from build123d import *

# Parameters (mm, degrees)
BOSS_EXTRUDE1_DEPTH = 9
FILLET1_R           = 3
FILLET2_R           = 2
CUT_EXTRUDE1_REACH  = 68.828
SKETCH2_R           = 2
DRAFT1_START        = 6.699702971
DRAFT1_OUTLINE_W    = 84
DRAFT1_OUTLINE_H    = 55
DRAFT1_DEPTH        = 4.532098623


# Read off the part's stored shape, not the designer's step: Draft1
with BuildPart() as part:
    # Sketch1 → Boss-Extrude1 (new body)
    # profile 1 of 4: a face of its own
    with BuildSketch(Plane(origin=(0, 0, 0), x_dir=(1, 0, 0), z_dir=(0, 1, 0))):
        Polygon((26, 26), (-26, 26), (-26, -22), (-41, -22), (-41, -26), (-26, -26), (26, -26), (41, -26), (41, -22), (26, -22), align=None)
        Polygon((-22, -19.632135629), (-22, 22), (-2.603209536, 22), (-1.5, 22), (-1.5, 19.632135629), (-1.5, -22), (-20.896790464, -22), (-22, -22), align=None, mode=Mode.SUBTRACT)
        Polygon((1.5, 19.632135629), (1.5, 22), (2.603209536, 22), (22, 22), (22, -19.632135629), (22, -22), (20.896790464, -22), (1.5, -22), align=None, mode=Mode.SUBTRACT)
    # profile 2 of 4: a face of its own
    with BuildSketch(Plane(origin=(0, 0, 0), x_dir=(1, 0, 0), z_dir=(0, 1, 0))):
        Polygon((26, 26), (-26, 26), (-26, -22), (-41, -22), (-41, -26), (-26, -26), (26, -26), (41, -26), (41, -22), (26, -22), align=None)
        Polygon((-22, -19.632135629), (-22, 22), (-2.603209536, 22), (-1.5, 22), (-1.5, 19.632135629), (-1.5, -22), (-20.896790464, -22), (-22, -22), align=None, mode=Mode.SUBTRACT)
        Polygon((1.5, 19.632135629), (1.5, 22), (2.603209536, 22), (22, 22), (22, -19.632135629), (22, -22), (20.896790464, -22), (1.5, -22), align=None, mode=Mode.SUBTRACT)
    # profile 3 of 4: a face of its own
    with BuildSketch(Plane(origin=(0, 0, 0), x_dir=(1, 0, 0), z_dir=(0, 1, 0))):
        Polygon((-1.5, 22), (-2.603209536, 22), (-22, -19.632135629), (-22, -22), (-20.896790464, -22), (-1.5, 19.632135629), align=None)
    # profile 4 of 4: a face of its own
    with BuildSketch(Plane(origin=(0, 0, 0), x_dir=(1, 0, 0), z_dir=(0, 1, 0))):
        Polygon((2.603209536, 22), (1.5, 22), (1.5, 19.632135629), (20.896790464, -22), (22, -22), (22, -19.632135629), align=None)
    extrude(amount=BOSS_EXTRUDE1_DEPTH)

    # Fillet1
    fillet1_edges = [part.edges().sort_by_distance(p)[0] for p in [
        (-26, 4.5, 22),
        (26, 4.5, 22),
        (22, 4.5, -22),
        (2.603209536, 4.5, -22),
        (-2.603209536, 4.5, -22),
        (-22, 4.5, -22),
        (20.896790464, 4.5, 22),
        (1.5, 4.5, 22),
        (-20.896790464, 4.5, 22),
        (-1.5, 4.5, 22),
    ]]
    fillet(fillet1_edges, radius=FILLET1_R)

    # Fillet2
    fillet2_edges = [part.edges().sort_by_distance(p)[0] for p in [
        (-26, 4.5, -26),
        (26, 4.5, -26),
        (41, 4.5, 26),
        (41, 4.5, 22),
        (-41, 4.5, 22),
        (-41, 4.5, 26),
    ]]
    fillet(fillet2_edges, radius=FILLET2_R - 0.0001)  # a hair under: the kernel refuses the full size

    # Sketch2 → Cut-Extrude1 (cut, up to next)
    with BuildSketch(Plane(origin=(0, 0, -26), x_dir=(-1, 0, 0), z_dir=(0, 0, -1)), mode=Mode.PRIVATE) as cut_extrude1_sk1:
        with Locations((-13, 4.5)):
            Circle(SKETCH2_R)
    cut_extrude1_tool1 = extrude(cut_extrude1_sk1.sketch, amount=-CUT_EXTRUDE1_REACH, mode=Mode.PRIVATE) & part.part
    # Sketch2 → Cut-Extrude1 (cut, up to next)
    with BuildSketch(Plane(origin=(0, 0, -26), x_dir=(-1, 0, 0), z_dir=(0, 0, -1)), mode=Mode.PRIVATE) as cut_extrude1_sk2:
        with Locations((13, 4.5)):
            Circle(SKETCH2_R)
    cut_extrude1_tool2 = extrude(cut_extrude1_sk2.sketch, amount=-CUT_EXTRUDE1_REACH, mode=Mode.PRIVATE) & part.part
    add(cut_extrude1_tool1.solids().sort_by_distance((13, 4.5, -26))[0], mode=Mode.SUBTRACT)
    add(cut_extrude1_tool2.solids().sort_by_distance((-13, 4.5, -26))[0], mode=Mode.SUBTRACT)

    # Draft1 outline → Draft1 (cut)
    with BuildSketch(Plane(origin=(0, 0, 0), x_dir=(1, 0, 0), z_dir=(0, 0.9961946980917455, 0.08715574274765815)).offset(DRAFT1_START)):
        with Locations((0, 0.5)):
            Rectangle(DRAFT1_OUTLINE_W, DRAFT1_OUTLINE_H)
    extrude(amount=DRAFT1_DEPTH, mode=Mode.SUBTRACT)


solid = part.part
Read the model definition and answer for the solid it produces. Units are mm, in the model's axes. A direction names the side the tool comes from. Give positions to 0.01 mm unless a question says otherwise; leave off trailing zeros. Write each loop counter-clockwise with the first axis right and the second up, starting at its lowest first coordinate (ties: lowest second). Pieces come first, ordered by that corner, then holes. Notation, with made-up numbers: (29.25, 56.5) - (68.25, 56.5) arc R32 ccw to (68.25, 89.5) - close; hole circle Ø9 at (73.25, -13). An arc over 180 degrees is marked (long way). Use CSV: the item, a comma, the result in double quotes. Start each with the question number.
Item 1: The part is cut by section C-C, the plane x = 2.5. Give the vertices of the cut face in (y, z), and give its area (3 significant figures).
Item 2: The mould has two halves that part along Z. Classify faces 1 (the cylindrical face through (26.9, 2.57, 21.14)), 2 (the flat face through (-26, 3, -3)), 3 (the cylindrical face through (-2.36, 2.57, 21.1)): pulls with the +Z half, pulls with the -Z half, needs draft (parallel to the pull), parting line crosses it, or undercut.
Item 3: Consider line 1 (Z direction, x = -18, y = 0.75); line 2 (X direction, y = 8, z = -15); line 3 (X direction, y = 1.5, z = 8.5). Determine where each line is inside the solid, lowest interval first.
Item 4: For faces 4 (the flat face through (26, 3, -2)), 5 (the flat face through (-34, 2, 22)), 6 (the flat face through (-1.5, 3, -1)), determine the directions among +Z, -Z, +X, -X, +Y, -Y from which every point of the face is accessible in a straight line to the end or side of a thin tool.
Item 5: Flat-ended cylindrical pins translate along their axes: P1, Ø4, axis at y = 3.5, z = -3, coming from the -X side; P2, Ø6, axis at x = 27.5, z = -0.5, coming from the +Y side; P3, Ø4, axis at y = 2.5, z = -6, coming from the +X side. Find the tip coordinate at first contact, or state that the pin passes through.
Item 6: The part is cut by section B-B, the plane x = 13. Give the vertices of the cut face in (y, z), and give its area (3 significant figures).
Item 7: The part is cut by section D-D, the plane z = 8.5. Give the vertices of the cut face in (x, y), and give its area (3 significant figures).
Item 8: The part is cut by section A-A, the plane z = -4.5. Give the vertices of the cut face in (x, y).
Taken from the geometry:
1,outline,"(0, -26) - (9, -26) - (8.26, -17.49) - (0, -17.49) - close; (0, 21.24) - (4.87, 21.24) - (4.45, 26) - (0, 26) - close"
1,area,"95.7 mm2"
2,face 1,"pulls with the -Z half"
2,face 2,"needs draft"
2,face 3,"undercut"
3,line 1,"-26 to -22, 11.05 to 15.78, 21.39 to 26"
3,line 2,"-26 to -22, -5.86 to -3.66, -1.5 to 1.5, 3.66 to 5.86, 22 to 26"
3,line 3,"-26 to -22, -16.81 to -14.61, -1.5 to 1.5, 14.61 to 16.81, 22 to 26"
4,face 4,"-Z, +X, +Y, -Y"
4,face 5,"-Z, -X, +Y, -Y"
4,face 6,"+Y, -Y"
5,P1,"x = -26"
5,P2,"y = 7"
5,P3,"x = 26"
6,outline,"(0, -26) - (2.5, -26) - (2.5, -22) - (0, -22) - close; (0, 0.32) - (6.7, 0.32) - (6.28, 5.05) - (0, 5.05) - close; (0, 22) - (4.8, 22) - (4.45, 26) - (0, 26) - close; (6.5, -26) - (9, -26) - (8.65, -22) - (6.5, -22) - close"
6,area,"68.5 mm2"
7,outline,"(-26, 0) - (-22, 0) - (-22, 5.98) - (-26, 5.98) - close; (-16.81, 0) - (-14.61, 0) - (-14.61, 5.98) - (-16.81, 5.98) - close; (-1.5, 0) - (1.5, 0) - (1.5, 5.98) - (-1.5, 5.98) - close; (14.61, 0) - (16.81, 0) - (16.81, 5.98) - (14.61, 5.98) - close; (22, 0) - (26, 0) - (26, 5.98) - (22, 5.98) - close"
7,area,"92.2 mm2"
8,outline,"(-26, 0) - (-22, 0) - (-22, 7.12) - (-26, 7.12) - close; (-10.76, 0) - (-8.55, 0) - (-8.55, 7.12) - (-10.76, 7.12) - close; (-1.5, 0) - (1.5, 0) - (1.5, 7.12) - (-1.5, 7.12) - close; (8.55, 0) - (10.76, 0) - (10.76, 7.12) - (8.55, 7.12) - close; (22, 0) - (26, 0) - (26, 7.12) - (22, 7.12) - close"
